Read the model definition and answer for the solid it produces. Units are mm, in the model's axes. Face numbers are marked on the shaded views. A direction names the side the tool comes from. Coordinates: 2 decimals unless noted, no trailing zeros. Order: outer loops, then holes, each group sorted by start corner. A loop starts at its lowest first (then second) coordinate and runs counter-clockwise, first axis right, second up. Notation, with made-up numbers: M -33,5.5 L -2,5.5 A18 cw -2,11.5 Z; hole C -13,27.25 d6. An arc over 180 degrees is marked long. Put each result on its own line as item: value.
Autodesk Inventor part; units mm, degrees
ref_plane "YZ Plane" through (0, 0, 0) normal (1, 0, 0) x (0, 1, 0)
ref_plane "XZ Plane" through (0, 0, 0) normal (0, 1, 0) x (-1, 0, 0)
ref_plane "XY Plane" through (0, 0, 0) normal (0, 0, 1) x (1, 0, 0)
sketch "Sketch1" plane through (0, 0, 0) normal (0, 0, 1) x (1, 0, 0)
  line L0 (0, 0) -> (10.16, 0)
  line L1 (10.16, 0) -> (10.16, 10.16)
  line L2 (10.16, 10.16) -> (0, 10.16)
  line L3 (0, 10.16) -> (0, 0)
  dimension "d0" = 10.16
  dimension "d1" = 10.16
extrude "Extrusion1" add sketch "Sketch1" along normal blind 6.985
sketch "Sketch2" plane through (0, 0, 6.985) normal (0, 0, 1) x (1, 0, 0)
  line L0 (0, 0) -> (10.16, 0) construction
  line L1 (10.16, 0) -> (10.16, 10.16) construction
  line L2 (10.16, 10.16) -> (0, 10.16) construction
  line L3 (0, 10.16) -> (0, 0) construction
  arc A0 (9.525, 10.16) -> (9.3363, 1.27) centre (16.3845, 5.5674) ccw
  arc A1 (7.3607, 10.16) -> (7.172, 1.27) centre (14.2202, 5.5674) ccw
  line L4 (7.3607, 10.16) -> (9.525, 10.16)
  line L5 (10.16, 10.16) -> (0, 10.16)
  line L6 (7.172, 1.27) -> (9.3363, 1.27)
  dimension "d4" = 8.255
  dimension "d5" = 0.635
  dimension "d6" = 1.27
extrude "Extrusion2" cut sketch "Sketch2" against normal blind 3.81
properties part number "limitSwitchTab" material "ABS Plastic"
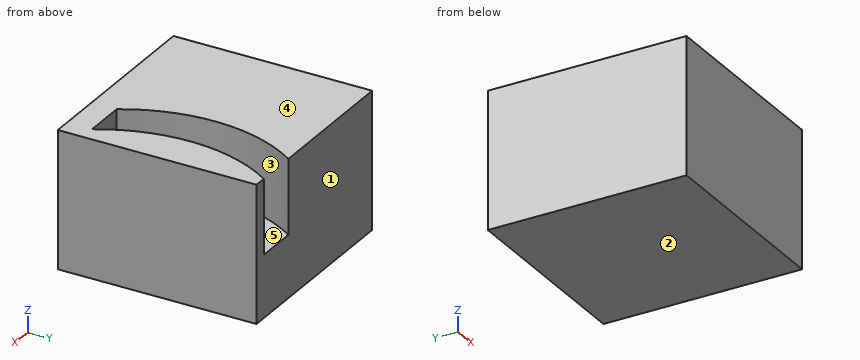
Q1. Consider line 1 along X through (y, z) = (5.5, 3.5); line 2 along Z through (x, y) = (7.75, 5.25) (3 decimals); line 3 along X through (y, z) = (8.75, 5). Determine where each line is inside the solid, lowest interval first.
Answers below:
line 1: x = 0 to 5.97, 8.13 to 10.16
line 2: z = 0 to 3.175
line 3: x = 0 to 6.6, 8.77 to 10.16
Q2. For a pull along Y with two mould halves and no side action, classify the marked faces 1, 2 and 3 as +Y half, -Y half, draft (parallel to the pull), parting line (faces both ways), or undercut.
Answers below:
face 1: +Y half
face 2: draft
face 3: undercut
Q3. Find section C-C on y = 7.5. Write down the section's boundary in (x, z) (3 decimals).
Answers below:
outline: M 0,0 L 10.16,0 L 10.16,6.985 L 8.359,6.985 L 8.359,3.175 L 6.195,3.175 L 6.195,6.985 L 0,6.985 Z
Q4. A tool of negligible diameter and unlimited length cuts with its end or side. For the marked faces 4 and 5, from which of +Z, -Z, +X, -X, +Y, -Y can it reach the whole face along a straight path? Write none if from no direction.
Answers below:
face 4: +Z, +X, -X, +Y, -Y
face 5: +Z
Q5. Find section B-B on x = 8. Write down the section's boundary in (y, z) (3 decimals).
Answers below:
outline: M 0,0 L 10.16,0 L 10.16,3.175 L 1.27,3.175 L 1.27,6.985 L 0,6.985 Z
Q6. Find section A-A on z = 6. Write down the section's boundary in (x, y) (3 decimals), plus the area to 3 significant figures.
Answers below:
outline: M 0,0 L 10.16,0 L 10.16,10.16 L 9.525,10.16 A8.255 ccw 9.336,1.27 L 7.172,1.27 A8.255 cw 7.361,10.16 L 0,10.16 Z
area: 84.0 mm^2
